Geometry check sheet. Reference: the model listing, model coordinates, mm. A direction names the side the tool comes from. Round coordinates to 2 decimals unless told otherwise and drop trailing zeros. Order: outer loops, then holes, each group sorted by start corner. A loop starts at its lowest first (then second) coordinate and runs counter-clockwise, first axis right, second up.
Autodesk Inventor part; units mm, degrees
ref_plane "YZ Plane" through (0, 0, 0) normal (1, 0, 0) x (0, 1, 0)
ref_plane "XZ Plane" through (0, 0, 0) normal (0, 1, 0) x (-1, 0, 0)
ref_plane "XY Plane" through (0, 0, 0) normal (0, 0, 1) x (1, 0, 0)
sketch "Sketch1" plane through (0, 0, 0) normal (0, 1, 0) x (-1, 0, 0)
  line L0 (0, 0) -> (44.45, 0)
  line L1 (44.45, 0) -> (44.45, 25.4)
  line L2 (44.45, 25.4) -> (261.62, 25.4)
  line L3 (261.62, 25.4) -> (261.62, 38.735)
  line L4 (261.62, 38.735) -> (0, 38.735)
  line L5 (0, 38.735) -> (0, 0)
  line L6 (0, 21.59) -> (38.1, 21.59)
  line L7 (38.1, 21.59) -> (38.1, 6.35)
  line L8 (38.1, 6.35) -> (0, 6.35)
  line L9 (0, 6.35) -> (0, 21.59)
  dimension "d9" = 44.45
  dimension "d10" = 25.4
  dimension "d17" = 261.62
  dimension "d24" = 38.735
  dimension "d26" = 15.24
  dimension "d27" = 6.35
  dimension "d50" = 217.17
  dimension "d51" = 6.35
extrude "Extrusion1" add sketch "Sketch1" along normal blind 19.05 contours L5 L8 L7 L6 L4 L3 L2 L1 L0
sketch "Sketch2" plane through (-261.62, 0, 38.735) normal (0, 0, 1) x (1, 0, 0)
  line L0 (261.62, 0) -> (261.62, 19.05)
  line L1 (0, 19.05) -> (261.62, 19.05)
  point P0 (247.65, 9.525)
  dimension "d37" = 13.97
  dimension "d38" = 19.05
  dimension "d39" = 9.525
hole "Hole1" at (-13.97, 9.525, 38.735) direction (0, 0, -1) diameter 12.827 end through all
sketch "Sketch3" plane through (-261.62, 0, 38.735) normal (0, 0, 1) x (1, 0, 0)
  line L0 (0, 0) -> (0, 19.05)
  line L1 (0, 19.05) -> (261.62, 19.05)
  point P0 (261.62, 0)
  point P1 (6.35, 9.525)
  dimension "d47" = 19.05
  dimension "d48" = 9.525
  dimension "d49" = 6.35
hole "Hole2" at (-255.27, 9.525, 38.735) direction (0, 0, -1) diameter 3.429 end through all
equation "\"d50\" = d17 - d9"
properties part number "shooter launch bar"
(1) Sectioned sample at D-D, the plane z = 11. Record the cut outline in (x, y).
Returned:
outline: (-44.45, 0) - (-38.1, 0) - (-38.1, 19.05) - (-44.45, 19.05) - close
(2) Set-up check for faces 4 (the flat face through (-152, 9, 25.4)), 5 (the flat face through (-22, 9, 0)), 6 (the flat face through (-23, 9, 21.59)): record each of +Z, -Z, +X, -X, +Y, -Y from which the full face is reachable in a straight line by a thin tool's end or side.
Returned:
face 4: -Z, -X, +Y, -Y
face 5: -Z, +X, -X, +Y, -Y
face 6: +X, +Y, -Y
(3) Depth check by flat-ended pin: P1, Ø5.5, axis at y = 13.5, z = 11.5, coming from the -X side; P2, Ø5.5, axis at x = -255.27, y = 9.525, coming from the -Z side; P3, Ø6, axis at y = 9.5, z = 10, coming from the +X side. Enter the tip coordinate at first touch or a pass-through.
Returned:
P1: stops at x = -44.45
P2: stops at z = 25.4
P3: stops at x = -38.1
(4) Sectioned sample at A-A, the plane x = -13.97. Give the number of separate pieces and of enclosed holes in the cut face, and give its area (3 significant figures).
Returned:
separate pieces: 4
enclosed holes: 0
area: 146 mm2
(5) Material ranges on line 1 (X direction, y = 9.5, z = 32.5); line 2 (Y direction, x = -13.97, z = 32); line 3 (Y direction, x = -255, z = 28), recorded low to high.
Returned:
line 1: x = -261.62 to -256.98, -253.56 to -20.38, -7.56 to 0
line 2: y = 0 to 3.11, 15.94 to 19.05
line 3: y = 0 to 7.83, 11.22 to 19.05
(6) Draft check along X on faces 1 (the cylindrical face through (-7.71, 10.92, 30.04)), 2 (the flat face through (-133, 9, 38.735)), 3 (the flat face through (-261.62, 9, 32)). Enter one of: released by +X, released by -X, zero draft, split by the parting line, or undercut.
Returned:
face 1: undercut
face 2: zero draft
face 3: released by -X
(7) Sectioned sample at C-C, the plane y = 13.5. Record the cut outline in (x, z) (3 decimals).
Returned:
outline: (-261.62, 25.4) - (-44.45, 25.4) - (-44.45, 0) - (-19.003, 0) - (-19.003, 6.35) - (-38.1, 6.35) - (-38.1, 21.59) - (-19.003, 21.59) - (-19.003, 38.735) - (-261.62, 38.735) - close; (-8.937, 0) - (0, 0) - (0, 6.35) - (-8.937, 6.35) - close; (-8.937, 21.59) - (0, 21.59) - (0, 38.735) - (-8.937, 38.735) - close
